The model under review builds one solid part; all positions refer to its coordinate system, in mm. Face numbers are marked on the shaded views. A direction names the side the tool comes from. Give positions to 0.01 mm unless a question says otherwise; leave off trailing zeros. Order: outer loops, then holes, each group sorted by start corner. A loop starts at its lowest first (then second) coordinate and runs counter-clockwise, first axis right, second up. Notation, with made-up numbers: (38.5, -10.75) - (80.5, -10.75) arc R18 ccw to (80.5, -1.75) - close; hole circle Ø10 at (55.5, -21). An arc over 180 degrees is marked (long way). Use CSV: the item, a comma, the result in double quotes. Start each with the question number.
1. Machinability: for the marked faces 1, 2 and 3, which of the approach directions +Z, -Z, +X, -X, +Y, -Y give a long, thin tool a straight path to every point of the face, cutting with its end or side? Answer none if there is none.
2. Take a section at B-B, the plane z = 17. State the section outline as (x, y) points.
3. Take a section at A-A, the plane x = 15. State the section outline as (y, z) points.
4. For pin 1 (0.9 mm diameter, centred on x = -8.5, z = 0, fed in from +Y); pin 2 (5 mm diameter, centred on x = 2, y = -120, fed in from +Z); pin 3 (8 mm diameter, centred on x = -5, z = 11, fed in from -Y); pin 4 (1.7 mm diameter, centred on x = -5.71, y = -150.24, fed in from -Z), all flat-tipped, find the tip position at first contact; note any pin that passes through.
5. To check wall thickness, follow line 1 (X direction, y = -154, z = -1.5); line 2 (Z direction, x = 8, y = -146.5); line 3 (Y direction, x = 13, z = 1.5). State the ranges of each line that lie inside material, in increasing order. Write a range as [from, to].
Autodesk Inventor part; units mm, degrees
ref_plane "YZ Plane" through (0, 0, 0) normal (1, 0, 0) x (0, 1, 0)
ref_plane "XZ Plane" through (0, 0, 0) normal (0, 1, 0) x (-1, 0, 0)
ref_plane "XY Plane" through (0, 0, 0) normal (0, 0, 1) x (1, 0, 0)
sketch "Sketch1" plane through (0, 0, 0) normal (1, 0, 0) x (0, 1, 0)
  circle A0 centre (-127.5274, 0) radius 19.939
  line L0 (-73.0444, 0) -> (-182.0104, 0) construction
  line L1 (-140.6798, 14.986) -> (-182.0104, 14.986)
  line L2 (-182.0104, -14.986) -> (-140.6798, -14.986)
  arc A1 (-182.0104, 14.986) -> (-182.0104, -14.986) centre (-182.0104, 0) ccw
  point P0 (0, 0)
  dimension "d0" = 39.878
  dimension "d1" = 29.972
  dimension "d2" = 89.408
extrude "Extrusion1" add sketch "Sketch1" along normal blind 25.019
sketch "Sketch2" plane through (0, 0, 0) normal (-1, 0, 0) x (0, 0, 1)
  line L0 (0.4128, -183.6614) -> (-0.4127, -183.6614)
  line L1 (-0.4127, -183.6614) -> (-0.4127, -178.3909)
  line L2 (-0.4127, -178.3909) -> (0.4128, -178.3909)
  line L3 (0.4128, -178.3909) -> (0.4128, -183.6614)
  line L4 (0.4128, -183.6614) -> (-0.4127, -178.3909) construction
  line L5 (-0.4127, -183.6614) -> (0.4128, -178.3909) construction
  line L6 (0.4128, -152.9909) -> (-0.4127, -152.9909)
  line L7 (-0.4127, -152.9909) -> (-0.4127, -147.7204)
  line L8 (-0.4127, -147.7204) -> (0.4128, -147.7204)
  line L9 (0.4128, -147.7204) -> (0.4128, -152.9909)
  line L10 (0.4128, -152.9909) -> (-0.4127, -147.7204) construction
  line L11 (-0.4127, -152.9909) -> (0.4128, -147.7204) construction
  arc A0 (14.986, -140.6798) -> (-14.986, -140.6798) centre (0, -127.5274) ccw
  line L12 (-14.986, -182.0104) -> (-14.986, -140.6798)
  arc A1 (-14.986, -182.0104) -> (14.986, -182.0104) centre (0, -182.0104) ccw
  line L13 (14.986, -140.6798) -> (14.986, -182.0104)
  point P0 (0, 0)
  point P1 (0, -181.0262)
  point P2 (0, -150.3557)
  point P3 (0, -150.3557)
  point P4 (0, -181.0262)
  point P5 (0, -150.3557)
  dimension "d5" = 5.2705
  dimension "d6" = 0.8255
  dimension "d7" = 40.132
  dimension "d8" = 25.4
extrude "Extrusion2" add sketch "Sketch2" along normal blind 11.8364 contours L0 L1 L2 L3 | L6 L7 L8 L9
sketch "Sketch3" plane through (0, -183.6614, -0.4127) normal (0, 0, -1) x (-1, 0, 0)
  circle A0 centre (9.8742, 2.7496) radius 1.124
  circle A1 centre (1.6192, 2.7496) radius 1.124
  circle A2 centre (5.7086, 2.7496) radius 0.7556
  circle A3 centre (1.6192, 33.42) radius 1.124
  circle A4 centre (5.7086, 33.42) radius 0.7556
  circle A5 centre (9.8742, 33.42) radius 1.124
  line L0 (0, 0) -> (0, 5.2705)
  line L1 (0, 0) -> (11.8364, 0)
  line L2 (11.8364, 5.2705) -> (11.8364, 0)
  line L3 (0, 5.2705) -> (11.8364, 5.2705)
  line L4 (0, 30.6705) -> (0, 35.941)
  line L5 (0, 30.6705) -> (11.8364, 30.6705)
  line L6 (11.8364, 35.941) -> (11.8364, 30.6705)
  line L7 (0, 35.941) -> (11.8364, 35.941)
  point P0 (0, 183.6614)
  dimension "d11" = 2.2479
  dimension "d12" = 1.6256
  dimension "d13" = 1.6256
  dimension "d14" = 0.8382
  dimension "d15" = 1.5113
  dimension "d16" = 2.286
  dimension "d17" = 2.2479
  dimension "d18" = 2.2098
extrude "Extrusion3" cut sketch "Sketch3" against normal through all contours A0 | A1 | A2 | A3 | A4 | A5
equation "\"d13\" = d12"
equation "\"d17\" = d11"
properties part number "OtherCamera"
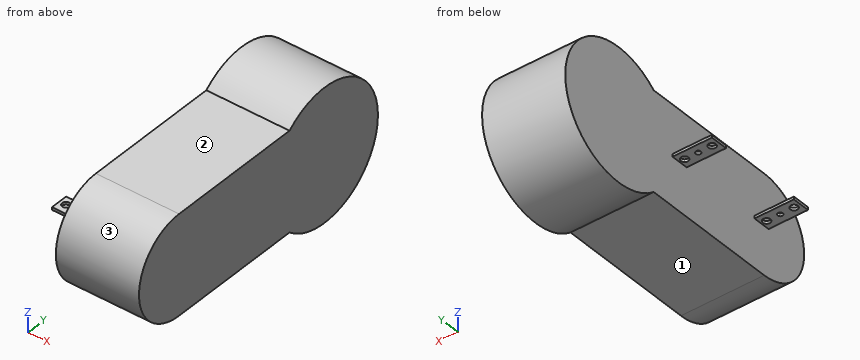
Determined:
1,face 1,"-Z, +X, -X, -Y"
1,face 2,"+Z, +X, -X, -Y"
1,face 3,"+X, -X, -Y"
2,outline,"(0, -137.95) - (25.02, -137.95) - (25.02, -117.11) - (0, -117.11) - close"
3,outline,"(-182.01, -14.99) - (-140.68, -14.99) arc R19.94 ccw (long way) to (-140.68, 14.99) - (-182.01, 14.99) arc R14.99 ccw to start"
4,pin 1,"stops at y = -147.72"
4,pin 2,"stops at z = 19.29"
4,pin 3,"passes through"
4,pin 4,"stops at z = -0.41"
5,line 1,"x = [0, 25.02]"
5,line 2,"z = [-14.99, 14.99]"
5,line 3,"y = [-196.92, -107.64]"
